from build123d import *

# Parameters (mm, degrees)
SKETCH1_W               = 46
SKETCH1_H               = 9
BOSS_EXTRUDE1_DEPTH     = 1
SKETCH2_W               = 1
SKETCH2_H               = 9
BOSS_EXTRUDE2_DEPTH     = 4
CUT_EXTRUDE1_DEPTH      = 47.489246068
CUT_EXTRUDE1_DEPTH_BACK = 47.489246068
SKETCH3_R               = 1
FILLET1_R               = 1
CUT_EXTRUDE2_DEPTH      = 4


with BuildPart() as part:
    # Sketch1 → Boss-Extrude1 (new body)
    with BuildSketch(Plane.XY):
        Rectangle(SKETCH1_W, SKETCH1_H)
    extrude(amount=BOSS_EXTRUDE1_DEPTH)

    # Sketch2 → Boss-Extrude2 (add)
    with BuildSketch(Plane.XY.offset(1)):
        with Locations((22.5, 0)):
            Rectangle(SKETCH2_W, SKETCH2_H)
        with Locations((-22.5, 0)):
            Rectangle(SKETCH2_W, SKETCH2_H)
    extrude(amount=BOSS_EXTRUDE2_DEPTH)

    # Sketch3 → Cut-Extrude1 (cut, two sides: drawn at the far end of the back side and taken through both)
    with BuildSketch(Plane(origin=(23, 0, 0), x_dir=(0, 0, -1), z_dir=(1, 0, 0)).offset(-CUT_EXTRUDE1_DEPTH_BACK)):
        with Locations((-2.519595735, 3.342695185)):
            Circle(SKETCH3_R)
        with Locations(Location((-2.519595735, -3.342695185, 0), (0, 0, 180))):
            Circle(SKETCH3_R)
    extrude(amount=CUT_EXTRUDE1_DEPTH + CUT_EXTRUDE1_DEPTH_BACK, mode=Mode.SUBTRACT)

    # Fillet1
    fillet1_edges = [part.edges().sort_by_distance(p)[0] for p in [
        (23, 0, 0),
        (-23, 0, 0),
    ]]
    fillet(fillet1_edges, radius=FILLET1_R)

    # Sketch4 → Cut-Extrude2 (cut)
    with BuildSketch(Plane(origin=(0, 0, 0), x_dir=(-1, 0, 0), z_dir=(0, 0, -1))):
        with BuildLine():
            Line((-13.969166326, 1.612266409), (13.969166326, 1.612266409))
            ThreePointArc((13.969166326, 1.612266409), (14.252009038, 1.729423696), (14.369166326, 2.012266409))
            Line((14.369166326, 2.012266409), (14.369166326, 2.564662734))
            ThreePointArc((14.369166326, 2.564662734), (14.252009038, 2.847505447), (13.969166326, 2.964662734))
            Line((13.969166326, 2.964662734), (-13.969166326, 2.964662734))
            ThreePointArc((-13.969166326, 2.964662734), (-14.252009038, 2.847505447), (-14.369166326, 2.564662734))
            Line((-14.369166326, 2.564662734), (-14.369166326, 2.012266409))
            ThreePointArc((-14.369166326, 2.012266409), (-14.252009038, 1.729423696), (-13.969166326, 1.612266409))
        make_face()
        with BuildLine():
            Line((14.369166326, -2.012266409), (14.369166326, -2.564662734))
            ThreePointArc((14.369166326, -2.564662734), (14.252009038, -2.847505447), (13.969166326, -2.964662734))
            Line((13.969166326, -2.964662734), (-13.969166326, -2.964662734))
            ThreePointArc((-13.969166326, -2.964662734), (-14.252009038, -2.847505447), (-14.369166326, -2.564662734))
            Line((-14.369166326, -2.564662734), (-14.369166326, -2.012266409))
            ThreePointArc((-14.369166326, -2.012266409), (-14.252009038, -1.729423696), (-13.969166326, -1.612266409))
            Line((-13.969166326, -1.612266409), (13.969166326, -1.612266409))
            ThreePointArc((13.969166326, -1.612266409), (14.252009038, -1.729423696), (14.369166326, -2.012266409))
        make_face()
        with BuildLine():
            Line((-21.6, 0.901467355), (-18.840541252, 0.901467355))
            ThreePointArc((-18.840541252, 0.901467355), (-18.55769854, 0.784310067), (-18.440541252, 0.501467355))
            Line((-18.440541252, 0.501467355), (-18.440541252, -0.615256763))
            ThreePointArc((-18.440541252, -0.615256763), (-18.55769854, -0.898099475), (-18.840541252, -1.015256763))
            Line((-18.840541252, -1.015256763), (-21.6, -1.015256763))
            ThreePointArc((-21.6, -1.015256763), (-21.882842712, -0.898099475), (-22, -0.615256763))
            Line((-22, -0.615256763), (-22, 0.501467355))
            ThreePointArc((-22, 0.501467355), (-21.882842712, 0.784310067), (-21.6, 0.901467355))
        make_face()
        with BuildLine():
            Line((18.440541252, 0.501467355), (18.440541252, -0.615256763))
            ThreePointArc((18.440541252, -0.615256763), (18.55769854, -0.898099475), (18.840541252, -1.015256763))
            Line((18.840541252, -1.015256763), (21.6, -1.015256763))
            ThreePointArc((21.6, -1.015256763), (21.882842712, -0.898099475), (22, -0.615256763))
            Line((22, -0.615256763), (22, 0.501467355))
            ThreePointArc((22, 0.501467355), (21.882842712, 0.784310067), (21.6, 0.901467355))
            Line((21.6, 0.901467355), (18.840541252, 0.901467355))
            ThreePointArc((18.840541252, 0.901467355), (18.55769854, 0.784310067), (18.440541252, 0.501467355))
        make_face()
    extrude(amount=-CUT_EXTRUDE2_DEPTH, mode=Mode.SUBTRACT)


solid = part.part
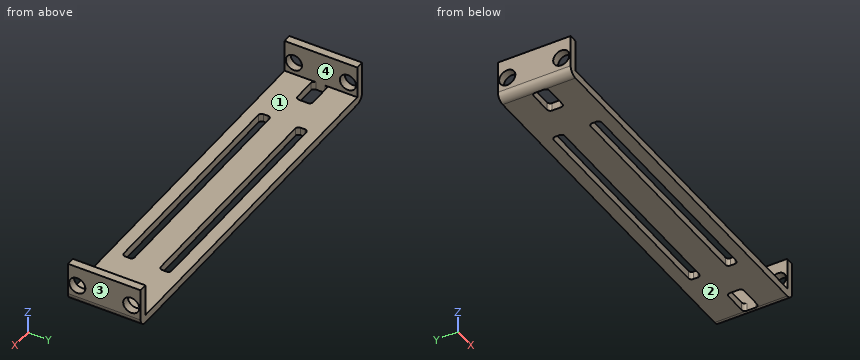
Could you check a few things on this model? Use its own coordinates, in mm. Face numbers are marked on the shaded views. Give positions to 0.01 mm unless a question says otherwise; leave off trailing zeros. Order: outer loops, then holes, each group sorted by start corner. A loop starts at its lowest first (then second) coordinate and runs counter-clockwise, first axis right, second up.
1. Suppose I cut it at A-A (x = -8). List the corners of the cut face in (y, z) for me, plus the area to 3 significant figures.
2. Will these pins go through, and if not, where does the flat tip stop? P1, Ø2, axis at x = 2, z = 2.5, coming from the +Y side; P2, Ø1, axis at x = -4, y = -1.5, coming from the +Z side; P3, Ø0.5, axis at y = 0, z = 0.5, coming from the +X side.
3. I need wall thicknesses on L1, parallel to Y at x = -6, z = 0.3; L2, parallel to X at y = -2.5, z = 4.85; L3, parallel to Y at x = -19.5, z = 0.7. Which ranges of each line are inside material? Lowest first, please.
4. Suppose I cut it at B-B (z = 3.95). List the corners of the cut face in (x, y) for me, plus the area to 3 significant figures.
5. We'd pull the mould along X, two halves only. Please class the marked faces 1, 2, 3 and 4: pulls with the +X half, pulls with the -X half, needs draft (parallel to the pull), parting line crosses it, or undercut.
Solved:
1. outline: (-4.5, 0) - (-2.96, 0) - (-2.96, 1) - (-4.5, 1) - close; (-1.61, 0) - (1.61, 0) - (1.61, 1) - (-1.61, 1) - close; (2.96, 0) - (4.5, 0) - (4.5, 1) - (2.96, 1) - close
1. area: 6.30 mm2
2. P1: passes through
2. P2: stops at z = 1
2. P3: stops at x = 22.97
3. L1: y = -4.5 to -2.96, -1.61 to 1.61, 2.96 to 4.5
3. L2: x = -23 to -22, 22 to 23
3. L3: y = -4.5 to -1.02, 0.9 to 4.5
4. outline: (-23, -4.5) - (-22, -4.5) - (-22, 4.5) - (-23, 4.5) - close; (22, -4.5) - (23, -4.5) - (23, 4.5) - (22, 4.5) - close
4. area: 18.0 mm2
5. face 1: undercut
5. face 2: needs draft
5. face 3: pulls with the +X half
5. face 4: undercut
